```python
from build123d import *

# Parameters (mm, degrees)
F1_DEPTH = 100
F2_W     = 30
F2_H     = 50
F3_DEPTH = 6
F4_R     = 1.5
F5_DEPTH = 8


with BuildPart() as f1:
    # F0 (on Right) → F1 (new body)
    with BuildSketch(Plane.YZ):
        Polygon((21.477706, -37.121146), (21.477706, 53.878854), (15.477706, 53.878854), (15.477706, -31.121146), (5.477706, -31.121146), (5.477706, -16.121146), (-0.522294, -16.121146), (-0.522294, -37.121146), align=None)
    extrude(amount=F1_DEPTH)

    # F2 (on face) → F3 (cut)
    with BuildSketch(Plane.XZ.offset(-15.477706)):
        with Locations((25, 13.878854)):
            Rectangle(F2_W, F2_H)
    extrude(amount=-F3_DEPTH, mode=Mode.SUBTRACT)

    # F4 (on face) → F5 (join)
    with BuildSketch(Plane.YZ.offset(100)):
        with Locations((18.477706, 43.878854)):
            Circle(F4_R)
        with Locations((18.477706, 23.878854)):
            Circle(F4_R)
        with Locations((18.477706, -7.121146)):
            Circle(F4_R)
        with Locations((18.477706, -27.121146)):
            Circle(F4_R)
    extrude(amount=F5_DEPTH)


solid = f1.part
```
Can you work these out from the model? Positions are in its coordinate system, mm. A direction names the side the tool comes from. Coordinates: 2 decimals unless noted, no trailing zeros. Loops run counter-clockwise (first coordinate to the right, second up) from the corner with the lowest first, then second, coordinate; pieces in that order, holes last. Notation, with made-up numbers: (-27.5, 11) -> (28.5, 11) arc R27 ccw to (28.5, 45) -> close; hole circle Ø3 at (46.5, 33.25). An arc over 180 degrees is marked (long way). Answer as a JSON object with one key per item and string values.
1) For P1, Ø6.5, axis at x = 36.5, y = 2.5, coming from the +Z side; P2, Ø3, axis at x = 68, y = 10, coming from the +Z side; P3, Ø3, axis at x = 86.5, z = 14.5, coming from the -Y side, each with a flat end and sliding along its axis, tell me the tip position at first contact or that it passes through.
Results:
{"P1": "stops at z = -16.12", "P2": "stops at z = -31.12", "P3": "stops at y = 15.48"}
2) For faces 1 (the face through (103.94, 19.86, -7.7)), 2 (the face through (108, 18, 24)), 3 (the face through (25, 18, -11.121)), 4 (the face through (49, 5.478, -24)), 5 (the face through (49, 3, -16.121)), which set-ups out of +Z, -Z, +X, -X, +Y, -Y let a thin tool reach every point of the face, with its end or its side?
Results:
{"face 1": "+X", "face 2": "+Z, -Z, +X, +Y, -Y", "face 3": "+Y, -Y", "face 4": "+Z, +X, -X", "face 5": "+Z, +X, -X, -Y"}
3) Imagine slicing it at B-B (z = 21). Please give me the cut outline in (x, y), then the cut area to 3 significant figures.
Results:
{"outline": "(0, 15.48) -> (10, 15.48) -> (10, 21.48) -> (0, 21.48) -> close; (40, 15.48) -> (100, 15.48) -> (100, 21.48) -> (40, 21.48) -> close", "area": "420 mm^2"}
4) Imagine slicing it at A-A (x = 30). Please give me the cut outline in (y, z), then the cut area to 3 significant figures.
Results:
{"outline": "(-0.52, -37.12) -> (21.48, -37.12) -> (21.48, -11.12) -> (15.48, -11.12) -> (15.48, -31.12) -> (5.48, -31.12) -> (5.48, -16.12) -> (-0.52, -16.12) -> close; (15.48, 38.88) -> (21.48, 38.88) -> (21.48, 53.88) -> (15.48, 53.88) -> close", "area": "432 mm^2"}
5) Imagine slicing it at C-C (x = 69.5). Please give me the cut outline in (y, z), then the cut area to 3 significant figures.
Results:
{"outline": "(-0.52, -37.12) -> (21.48, -37.12) -> (21.48, 53.88) -> (15.48, 53.88) -> (15.48, -31.12) -> (5.48, -31.12) -> (5.48, -16.12) -> (-0.52, -16.12) -> close", "area": "732 mm^2"}
6) Imagine slicing it at D-D (y = 12.75). Please give me the cut outline in (x, z), then the cut area to 3 significant figures.
Results:
{"outline": "(0, -37.12) -> (100, -37.12) -> (100, -31.12) -> (0, -31.12) -> close", "area": "600 mm^2"}
7) If I drill on line 1 (X direction, y = 18.25, z = 35.5); line 2 (Z direction, x = 63, y = 8.5); line 3 (X direction, y = 1.75, z = -19), over which ranges is the centre line in solid material (lowest first)?
Results:
{"line 1": "x = 0 to 10, 40 to 100", "line 2": "z = -37.12 to -31.12", "line 3": "x = 0 to 100"}
8) Thinking about a two-plate mould opening in Z: for faces 6 (the face through (40, 18, 14)), 7 (the face through (49, 11, -31.121)), 8 (the face through (108, 18, -27)), 9 (the face through (103.94, 19.91, 24.33)), which applies, pulls with the +Z half, pulls with the -Z half, needs draft (parallel to the pull), parting line crosses it, or undercut?
Results:
{"face 6": "undercut", "face 7": "pulls with the +Z half", "face 8": "needs draft", "face 9": "undercut"}
